from build123d import *

# Parameters (mm, degrees)
PAD_DEPTH       = 1.8
SKETCH001_R     = 3
PAD001_DEPTH    = 1.7
SKETCH002_R     = 2.5
PAD002_DEPTH    = 1
SKETCH003_R     = 2
POCKET_DEPTH    = 1.4
SKETCH004_R     = 2.35
POCKET001_DEPTH = 2.5
SKETCH005_R     = 1.35
POCKET002_DEPTH = 4.501
SKETCH006_R     = 0.5
POCKET003_DEPTH = 2.801


with BuildPart() as part:
    # Sketch → Pad (new body)
    with BuildSketch(Plane.XY):
        with BuildLine():
            ThreePointArc((0.2238838654, 2.9916343384), (-3, -2.741e-07), (0.223884412, -2.9916342975))
            Line((13.5492701682, -1.9944218252), (0.223884412, -2.9916342975))
            ThreePointArc((13.5492701681, -1.9944218252), (15.4, 0), (13.5492701681, 1.9944218252))
            Line((13.5492701682, 1.9944218252), (0.2238838654, 2.9916343384))
        make_face()
    extrude(amount=PAD_DEPTH)

    # Sketch001 → Pad001 (new body)
    with BuildSketch(Plane.XY.offset(1.8)):
        Circle(SKETCH001_R)
    extrude(amount=PAD001_DEPTH)

    # Sketch002 → Pad002 (new body)
    with BuildSketch(Plane(origin=(0, 0, 0), x_dir=(1, 0, 0), z_dir=(0, 0, -1))):
        Circle(SKETCH002_R)
    extrude(amount=PAD002_DEPTH)

    # Sketch003 → Pocket (cut)
    with BuildSketch(Plane(origin=(0, 0, -1), x_dir=(1, 0, 0), z_dir=(0, 0, -1))):
        Circle(SKETCH003_R)
    extrude(amount=-POCKET_DEPTH, mode=Mode.SUBTRACT)

    # Sketch004 → Pocket001 (cut)
    with BuildSketch(Plane.XY.offset(3.5)):
        Circle(SKETCH004_R)
    extrude(amount=-POCKET001_DEPTH, mode=Mode.SUBTRACT)

    # Sketch005 → Pocket002 (cut, through all)
    with BuildSketch(Plane.XY.offset(3.5)):
        Circle(SKETCH005_R)
    extrude(amount=-POCKET002_DEPTH, mode=Mode.SUBTRACT)

    # Sketch006 → Pocket003 (cut, through all)
    with BuildSketch(Plane.XY.offset(1.8)):
        with Locations((7.3, 0)):
            Circle(SKETCH006_R)
        with Locations((10.3, 0)):
            Circle(SKETCH006_R)
        with Locations((13.3, 0)):
            Circle(SKETCH006_R)
    extrude(amount=-POCKET003_DEPTH, mode=Mode.SUBTRACT)


solid = part.part
Design review of the part built by this model. Coordinates are the model's own, in mm. A direction names the side the tool comes from. Coordinates: 2 decimals unless noted, no trailing zeros. Write each loop counter-clockwise with the first axis right and the second up, starting at its lowest first coordinate (ties: lowest second). Pieces come first, ordered by that corner, then holes. Notation, with made-up numbers: (36, 76.5) - (54, 76.5) arc R11 cw to (54, 85.5) - close; hole circle Ø4 at (-8.5, 28). An arc over 180 degrees is marked (long way). One line per item, written item: value.
1) To check wall thickness, follow probe 1 along Y at (x, z) = (0, -0.2); probe 2 along Y at (x, z) = (0, 2.65). State the ranges of each line that lie inside material, in increasing order.
Answer sheet:
probe 1: y = -2.5 to -2, 2 to 2.5
probe 2: y = -3 to -2.35, 2.35 to 3
2) Add section C-C (z = 0.6). State the section outline as (x, y) points.
Answer sheet:
outline: (0.22, -2.99) - (13.55, -1.99) arc R2 ccw to (13.55, 1.99) - (0.22, 2.99) arc R3 ccw (long way) to start; hole circle Ø2.7 at (0, 0); hole circle Ø1 at (7.3, 0); hole circle Ø1 at (10.3, 0); hole circle Ø1 at (13.3, 0)
3) For faces 1 (the face through (0, -2, 1)), 2 (the face through (15.4, 0, 0.9)), 3 (the face through (-0.54, 2.44, -0.49)), list the 3-axis set-ups (+Z, -Z, +X, -X, +Y, -Y) from which the entire face can be reached by the end or side of a thin tool; tool diameter is ignored.
Answer sheet:
face 1: +Z
face 2: +Z, -Z, +X
face 3: -Z
4) Insertion check: pin 1 (3 mm diameter, centred on x = 0, y = 0, fed in from +Z); pin 2 (2 mm diameter, centred on x = -0.5, y = 0, fed in from -Z); pin 3 (2 mm diameter, centred on x = 3, z = 2.5, fed in from -Y). Each pin has a flat end and moves straight along its axis. Give the tip position at first contact, or say it passes through.
Answer sheet:
pin 1: stops at z = 1
pin 2: stops at z = 0.4
pin 3: stops at y = -2.84
5) Add section D-D (y = -0.8). State the section outline as (x, z) points.
Answer sheet:
outline: (-2.89, 0) - (-2.37, 0) - (-2.37, -1) - (-1.83, -1) - (-1.83, 0.4) - (-1.09, 0.4) - (-1.09, 1) - (-2.21, 1) - (-2.21, 3.5) - (-2.89, 3.5) - close; (1.09, 0.4) - (1.83, 0.4) - (1.83, -1) - (2.37, -1) - (2.37, 0) - (15.23, 0) - (15.23, 1.8) - (2.89, 1.8) - (2.89, 3.5) - (2.21, 3.5) - (2.21, 1) - (1.09, 1) - close
6) Add section A-A (x = 0). State the section outline as (y, z) points.
Answer sheet:
outline: (-3, 0) - (-2.5, 0) - (-2.5, -1) - (-2, -1) - (-2, 0.4) - (-1.35, 0.4) - (-1.35, 1) - (-2.35, 1) - (-2.35, 3.5) - (-3, 3.5) - close; (1.35, 0.4) - (2, 0.4) - (2, -1) - (2.5, -1) - (2.5, 0) - (3, 0) - (3, 3.5) - (2.35, 3.5) - (2.35, 1) - (1.35, 1) - close
7) Add section B-B (y = 0). Give the number of separate pieces and of enclosed holes in the cut face, plus the area to 4 significant figures.
Answer sheet:
separate pieces: 5
enclosed holes: 0
area: 23.95 mm2
